```python
from build123d import *

# Parameters (mm, degrees)
SKETCH_1_W      = 50
SKETCH_1_H      = 150
SKETCH_1_R      = 1.3
EXTRUDE_1_DEPTH = 4
SKETCH_3_W      = 27
SKETCH_3_H      = 62.5
EXTRUDE_2_DEPTH = 3
FILLET_1_R      = 5


with BuildPart() as part:
    # 草图1 → 凸台-拉伸1 (new body)
    with BuildSketch(Plane(origin=(0, 0, 0), x_dir=(1, 0, 0), z_dir=(0, 1, 0))):
        Rectangle(SKETCH_1_W, SKETCH_1_H)
        with Locations(Location((0, 7.25, 0), (0, 0, 270))):
            Circle(SKETCH_1_R, mode=Mode.SUBTRACT)
        with Locations(Location((0, -7.25, 0), (0, 0, 270))):
            Circle(SKETCH_1_R, mode=Mode.SUBTRACT)
        with Locations(Location((-18.5, 0, 0), (0, 0, 270))):
            Circle(SKETCH_1_R, mode=Mode.SUBTRACT)
        with Locations(Location((18.5, 0, 0), (0, 0, 270))):
            Circle(SKETCH_1_R, mode=Mode.SUBTRACT)
        with Locations(Location((-16, -40, 0), (0, 0, 270))):
            Circle(SKETCH_1_R, mode=Mode.SUBTRACT)
        with Locations(Location((16, -40, 0), (0, 0, 270))):
            Circle(SKETCH_1_R, mode=Mode.SUBTRACT)
        with Locations(Location((-16, -60, 0), (0, 0, 270))):
            Circle(SKETCH_1_R, mode=Mode.SUBTRACT)
        with Locations(Location((16, -60, 0), (0, 0, 270))):
            Circle(SKETCH_1_R, mode=Mode.SUBTRACT)
        with Locations(Location((-16, 40, 0), (0, 0, 270))):
            Circle(SKETCH_1_R, mode=Mode.SUBTRACT)
        with Locations(Location((16, 40, 0), (0, 0, 270))):
            Circle(SKETCH_1_R, mode=Mode.SUBTRACT)
        with Locations(Location((-16, 60, 0), (0, 0, 270))):
            Circle(SKETCH_1_R, mode=Mode.SUBTRACT)
        with Locations(Location((16, 60, 0), (0, 0, 270))):
            Circle(SKETCH_1_R, mode=Mode.SUBTRACT)
    extrude(amount=EXTRUDE_1_DEPTH)

    # 草图3 → 凸台-拉伸2 (add)
    with BuildSketch(Plane.XZ):
        with Locations((0, 43.75)):
            Rectangle(SKETCH_3_W, SKETCH_3_H)
        with Locations((0, -43.75)):
            Rectangle(SKETCH_3_W, SKETCH_3_H)
    extrude(amount=EXTRUDE_2_DEPTH)

    # 圆角1
    fillet_1_edges = [part.edges().sort_by_distance(p)[0] for p in [
        (25, 2, 75),
        (-25, 2, 75),
        (-25, 2, -75),
        (25, 2, -75),
    ]]
    fillet(fillet_1_edges, radius=FILLET_1_R)


solid = part.part
```
Can you work these out from the model? Positions are in its coordinate system, mm. A direction names the side the tool comes from. Coordinates: 2 decimals unless noted, no trailing zeros. Loops run counter-clockwise (first coordinate to the right, second up) from the corner with the lowest first, then second, coordinate; pieces in that order, holes last. Notation, with made-up numbers: M 20.25,-17.75 L 31.25,-17.75 A23 ccw 31.25,4.25 Z; hole C 71,24 d3. An arc over 180 degrees is marked long. Put each result on its own line as item: value. Start each with the question number.
(1) We'd pull the mould along Z, two halves only. Please class faces 1 (the face through (25, 2, 1)), 2 (the face through (-15.94, 1.97, 38.7)), 3 (the face through (-24, 2, -73)), 4 (the face through (0.39, 1.97, 8.49)): +Z half, -Z half, draft (parallel to the pull), parting line (faces both ways), or undercut.
(2) Imagine slicing it at A-A on z = 0. List the corners of the cut face in (x, y) for me, and give its area (3 significant figures).
(3) Imagine slicing it at B-B on z = -45. List the corners of the cut face in (x, y) for me, and give its area (3 significant figures).
(4) Imagine slicing it at C-C on x = 5. List the corners of the cut face in (y, z) for me, and give its area (3 significant figures).
(5) I need wall thicknesses on probe 1 along X at (y, z) = (1.75, 60); probe 2 along Z at (x, y) = (-6.5, -2.25); probe 3 along X at (y, z) = (2.6, -7.25). Which ranges of each line are inside material? Lowest first, please.
(6) Will these pins go through, and if not, where does the flat tip stop? pin 1 Ø3 at (x, z) = (16, -60) entering from -Y; pin 2 Ø2.5 at (x, z) = (16, 40) entering from +Y; pin 3 Ø2.5 at (y, z) = (-2, -47.5) entering from -X.
(7) Imagine slicing it at D-D on z = 40. List the corners of the cut face in (x, y) for me.
(8) Which directions (+Z, -Z, +X, -X, +Y, -Y) give clear straight access to the entire face, cutting with the end or side of a thin tool? Please do faces 5 (the face through (17.23, 1.97, -0.28)), 6 (the face through (-13.5, -1, -44)), 7 (the face through (-24, 2, 73)), 8 (the face through (0, -1, 12.5)), 9 (the face through (13.5, -1, -44)).
Worked answers:
1. face 1: draft
1. face 2: undercut
1. face 3: -Z half
1. face 4: undercut
2. outline: M -25,0 L -19.8,0 L -19.8,4 L -25,4 Z; M -17.2,0 L 17.2,0 L 17.2,4 L -17.2,4 Z; M 19.8,0 L 25,0 L 25,4 L 19.8,4 Z
2. area: 179 mm2
3. outline: M -25,0 L -13.5,0 L -13.5,-3 L 13.5,-3 L 13.5,0 L 25,0 L 25,4 L -25,4 Z
3. area: 281 mm2
4. outline: M -3,-75 L 4,-75 L 4,75 L -3,75 L -3,12.5 L 0,12.5 L 0,-12.5 L -3,-12.5 Z
4. area: 975 mm2
5. probe 1: x = -25 to -17.3, -14.7 to 14.7, 17.3 to 25
5. probe 2: z = -75 to -12.5, 12.5 to 75
5. probe 3: x = -25 to -1.3, 1.3 to 25
6. pin 1: stops at y = 0
6. pin 2: passes through
6. pin 3: stops at x = -13.5
7. outline: M -25,0 L -17.3,0 L -17.3,4 L -25,4 Z; M -14.7,0 L -13.5,0 L -13.5,-3 L 13.5,-3 L 13.5,0 L 14.7,0 L 14.7,4 L -14.7,4 Z; M 17.3,0 L 25,0 L 25,4 L 17.3,4 Z
8. face 5: +Y, -Y
8. face 6: +Z, -Z, -X, -Y
8. face 7: +Z, -X, +Y, -Y
8. face 8: +X, -X, -Y
8. face 9: +Z, -Z, +X, -Y
